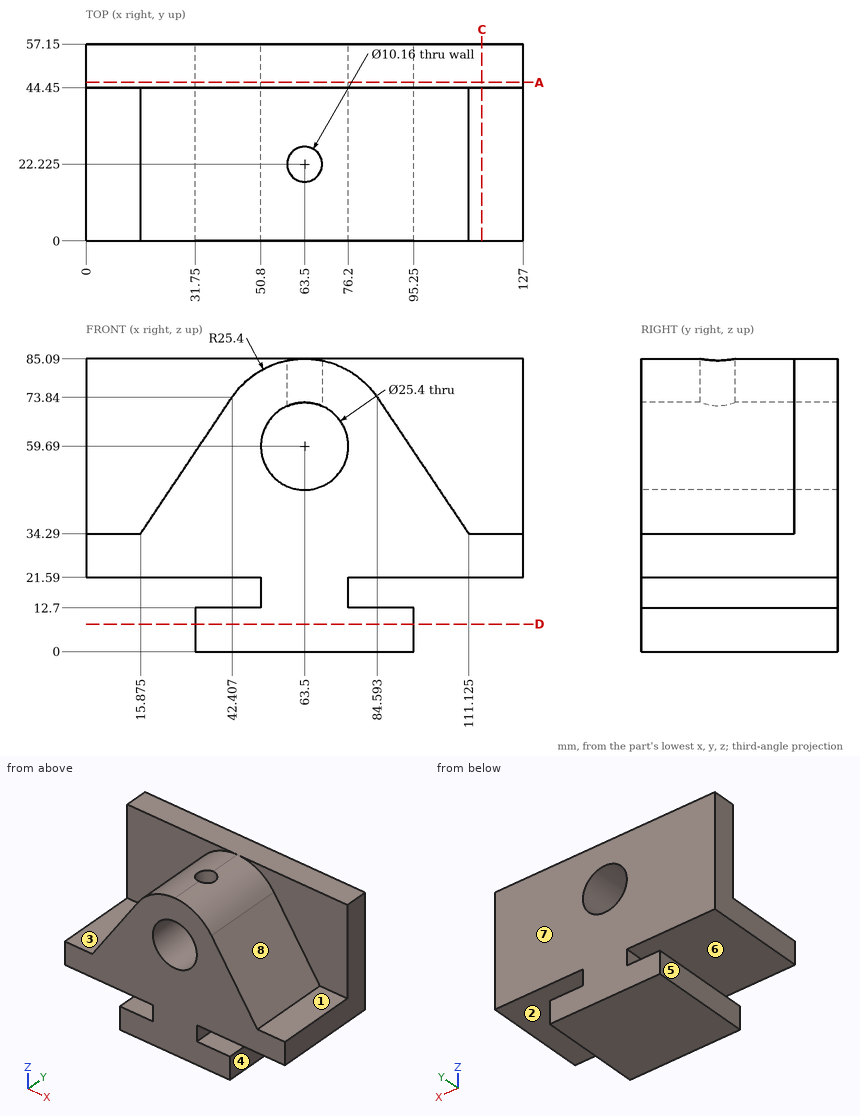
Part print with two shaded views. Sizes in mm from the minimum x, y, z corner. A direction names the side the tool comes from. Round coordinates to 2 decimals unless told otherwise and drop trailing zeros. Write each loop counter-clockwise with the first axis right and the second up, starting at its lowest first coordinate (ties: lowest second). Pieces come first, ordered by that corner, then holes. Notation, with made-up numbers: (-28.75, 46) -> (-11.75, 46) arc R25 cw to (-11.75, 81) -> close; hole circle Ø9 at (77.25, -18). An arc over 180 degrees is marked (long way). Put each result on its own line as item: value.
Item 1: Slice it at C-C, the plane x = 115. Give the cut face in (y, z), plus the area to 3 significant figures.
Here are the results:
outline: (0, 21.59) -> (57.15, 21.59) -> (57.15, 85.09) -> (44.45, 85.09) -> (44.45, 34.29) -> (0, 34.29) -> close
area: 1,370 mm^2
Item 2: Slice it at D-D, the plane z = 8. Give the cut face in (x, y).
Here are the results:
outline: (31.75, 0) -> (95.25, 0) -> (95.25, 57.15) -> (31.75, 57.15) -> close
Item 3: Slice it at A-A, the plane y = 46. Give the cut face in (x, z).
Here are the results:
outline: (0, 21.59) -> (50.8, 21.59) -> (50.8, 12.7) -> (31.75, 12.7) -> (31.75, 0) -> (95.25, 0) -> (95.25, 12.7) -> (76.2, 12.7) -> (76.2, 21.59) -> (127, 21.59) -> (127, 85.09) -> (0, 85.09) -> close; hole circle Ø25.4 at (63.5, 59.69)
Item 4: Tool access for the marked faces 1, 2, 3, 4 and 5: list every direction of +Z, -Z, +X, -X, +Y, -Y with a clear straight run to the whole face (end or side of a thin tool).
Here are the results:
face 1: +Z, +X, -Y
face 2: +X, +Y, -Y
face 3: +Z, -X, -Y
face 4: -Z, +X, +Y, -Y
face 5: -Z, -X, +Y, -Y
Item 5: Two-plate mould, pull along Z, no slides. Class the marked faces 6, 7 and 8: pulls with the +Z half, pulls with the -Z half, needs draft (parallel to the pull), parting line crosses it, or undercut.
Here are the results:
face 6: undercut
face 7: needs draft
face 8: pulls with the +Z half
Item 6: Wall check: probe 1 along Z at (x, y) = (93, 53.5); probe 2 along Z at (x, y) = (63, 18); probe 3 along Y at (x, z) = (94.5, 81). Give the ranges that are in metal, low to high. Write a range as from..to.
Here are the results:
probe 1: z = 0..12.7, 21.59..85.09
probe 2: z = 0..47
probe 3: y = 44.45..57.15
Item 7: Flat gauge pins, fed straight in: P1, Ø4, axis at y = 35.5, z = 4.5, coming from the -X side; P2, Ø4, axis at x = 21, y = 15.5, coming from the +Z side; P3, Ø9.5, axis at x = 83.5, y = 23, coming from the +Z side. Where does each tip first touch, or does it go through?
Here are the results:
P1: stops at x = 31.75
P2: stops at z = 44.91
P3: stops at z = 80
